Print and shaded views of the part. All mm, measured from the part's lowest x, y and z. Give positions to 0.01 mm unless a question says otherwise; leave off trailing zeros. Write each loop counter-clockwise with the first axis right and the second up, starting at its lowest first coordinate (ties: lowest second). Pieces come first, ordered by that corner, then holes. Notation, with made-up numbers: (51.5, 32.5) - (86.5, 32.5) arc R22 cw to (86.5, 45.5) - close; hole circle Ø11 at (23, -32). An arc over 180 degrees is marked (long way). Use one line per item in the form item = value. Start each with the question number.
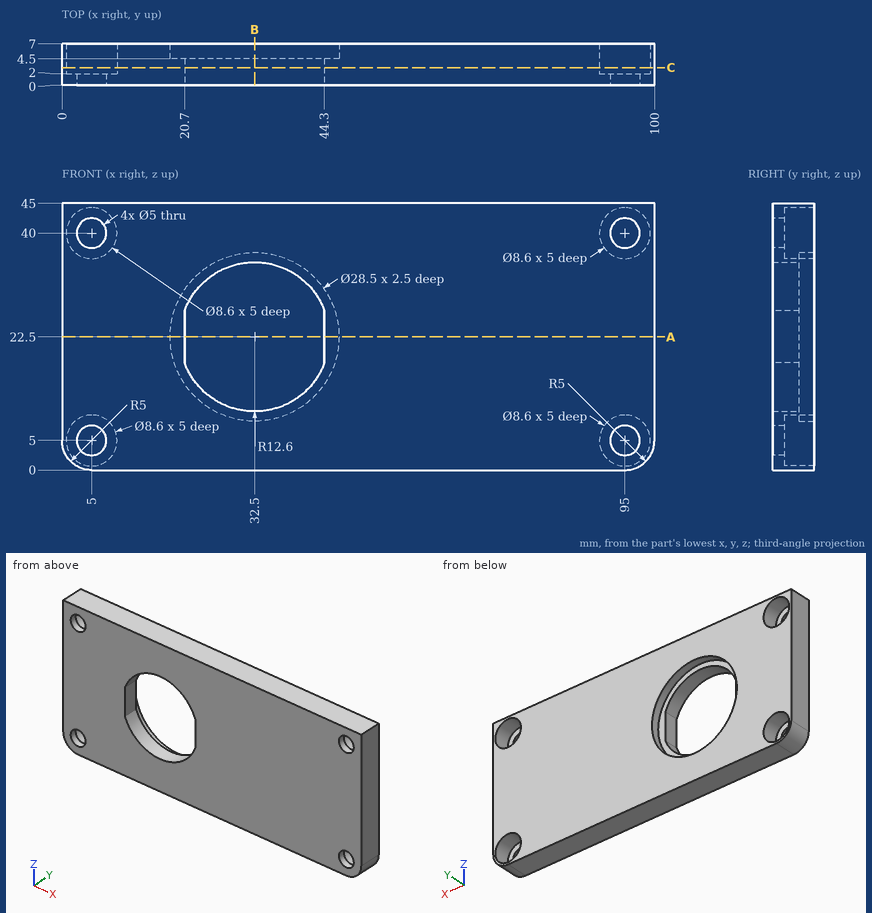
(1) Pin check, flat tip, straight feed: pin 1 Ø6 at (x, z) = (5, 5) entering from +Y. Stop position of the tip, or through.
(2) Cut at B-B, the plane x = 32.5. Give the cut face in (y, z).
(3) Cut at A-A, the plane z = 22.5. Give the cut face in (x, y), then the cut area to 3 significant figures.
(4) Wall check: line 1 (X direction, y = 1.6, z = 40); line 2 (Z direction, x = 95, y = 4.15); line 3 (Z direction, x = 5, y = 0.8). Give the ranges that are in metal, low to high. Write a range as from..to.
(5) Cut at C-C, the plane y = 3. Give the cut face in (x, z), then the cut area to 3 significant figures.
Solution:
q1.pin_1 = 2
q2.outline = (0, 0) - (7, 0) - (7, 8.25) - (4.5, 8.25) - (4.5, 9.9) - (0, 9.9) - close; (0, 35.1) - (4.5, 35.1) - (4.5, 36.75) - (7, 36.75) - (7, 45) - (0, 45) - close
q3.outline = (0, 0) - (20.7, 0) - (20.7, 4.5) - (18.25, 4.5) - (18.25, 7) - (0, 7) - close; (44.3, 0) - (100, 0) - (100, 7) - (46.75, 7) - (46.75, 4.5) - (44.3, 4.5) - close
q3.area = 523 mm2
q4.line_1 = 0..2.5, 7.5..92.5, 97.5..100
q4.line_2 = 0..0.7, 9.3..35.7, 44.3..45
q4.line_3 = 0..2.5, 7.5..37.5, 42.5..45
q5.outline = (0, 5) arc R5 ccw to (5, 0) - (95, 0) arc R5 ccw to (100, 5) - (100, 45) - (0, 45) - close; hole circle Ø8.6 at (5, 5); hole circle Ø8.6 at (5, 40); hole (20.7, 18.08) arc R12.6 ccw to (44.3, 18.08) - (44.3, 26.92) arc R12.6 ccw to (20.7, 26.92) - close; hole circle Ø8.6 at (95, 5); hole circle Ø8.6 at (95, 40)
q5.area = 3,770 mm2
